The figure shows three views and two pictorial views of one solid part (mm, origin at its lowest corner). Answer the questions. A direction names the side the tool comes from. Coordinates: 2 decimals unless noted, no trailing zeros. Order: outer loops, then holes, each group sorted by start corner. A loop starts at its lowest first (then second) coordinate and runs counter-clockwise, first axis right, second up. Notation, with made-up numbers: (-3, -21) -> (37, -21) arc R20 cw to (37, -6) -> close; hole circle Ø8 at (88, 72). An arc over 180 degrees is marked (long way). Return JSON: item names as keys, results as strings.
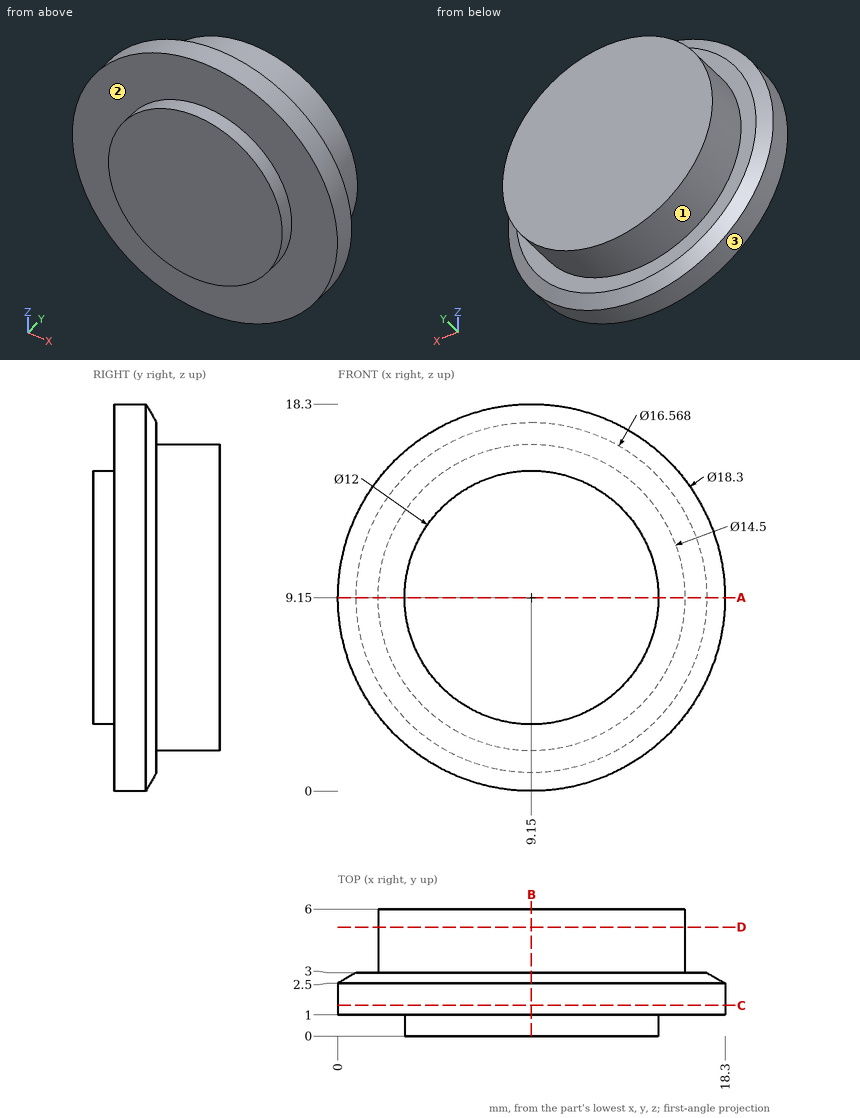
Item 1: The part is cut by section D-D on y = 5.15. Determine the outline of the cut face in (x, z), plus the area to 3 significant figures.
Answer list:
{"outline": "circle Ø14.5 at (9.15, 9.15)", "area": "165 mm2"}
Item 2: Which of the six approach directions +Z, -Z, +X, -X, +Y, -Y give full straight-line access (tool end or side, diameter ignored) to the marked faces 1, 2 and 3?
Answer list:
{"face 1": "+Y", "face 2": "-Y", "face 3": "+Y, -Y"}
Item 3: The part is cut by section C-C on y = 1.45. Determine the outline of the cut face in (x, z).
Answer list:
{"outline": "circle Ø18.3 at (9.15, 9.15)"}
Item 4: The part is cut by section A-A on z = 9.15. Determine the outline of the cut face in (x, y), plus the area to 3 significant figures.
Answer list:
{"outline": "(0, 1) -> (3.15, 1) -> (3.15, 0) -> (15.15, 0) -> (15.15, 1) -> (18.3, 1) -> (18.3, 2.5) -> (17.43, 3) -> (16.4, 3) -> (16.4, 6) -> (1.9, 6) -> (1.9, 3) -> (0.87, 3) -> (0, 2.5) -> close", "area": "91.7 mm2"}
Item 5: A flat-ended cylindrical pin translates along its axis: pin 1 (3 mm diameter, centred on x = 11, y = 1.5, fed in from -Z). Find the tip coordinate at first contact, or state that the pin passes through.
Answer list:
{"pin 1": "z = 0.01"}
Item 6: The part is cut by section B-B on x = 9.15. Determine the outline of the cut face in (y, z), plus the area to 3 significant figures.
Answer list:
{"outline": "(0, 3.15) -> (1, 3.15) -> (1, 0) -> (2.5, 0) -> (3, 0.87) -> (3, 1.9) -> (6, 1.9) -> (6, 16.4) -> (3, 16.4) -> (3, 17.43) -> (2.5, 18.3) -> (1, 18.3) -> (1, 15.15) -> (0, 15.15) -> close", "area": "91.7 mm2"}
Item 7: Find the intervals of material crossed by probe 1 along Y at (x, z) = (13, 16.25); probe 2 along Z at (x, y) = (2.5, 1.8) (3 decimals); probe 3 along X at (y, z) = (4.55, 15), in increasing order.
Answer list:
{"probe 1": "1 to 3", "probe 2": "2.865 to 15.435", "probe 3": "4.87 to 13.43"}
